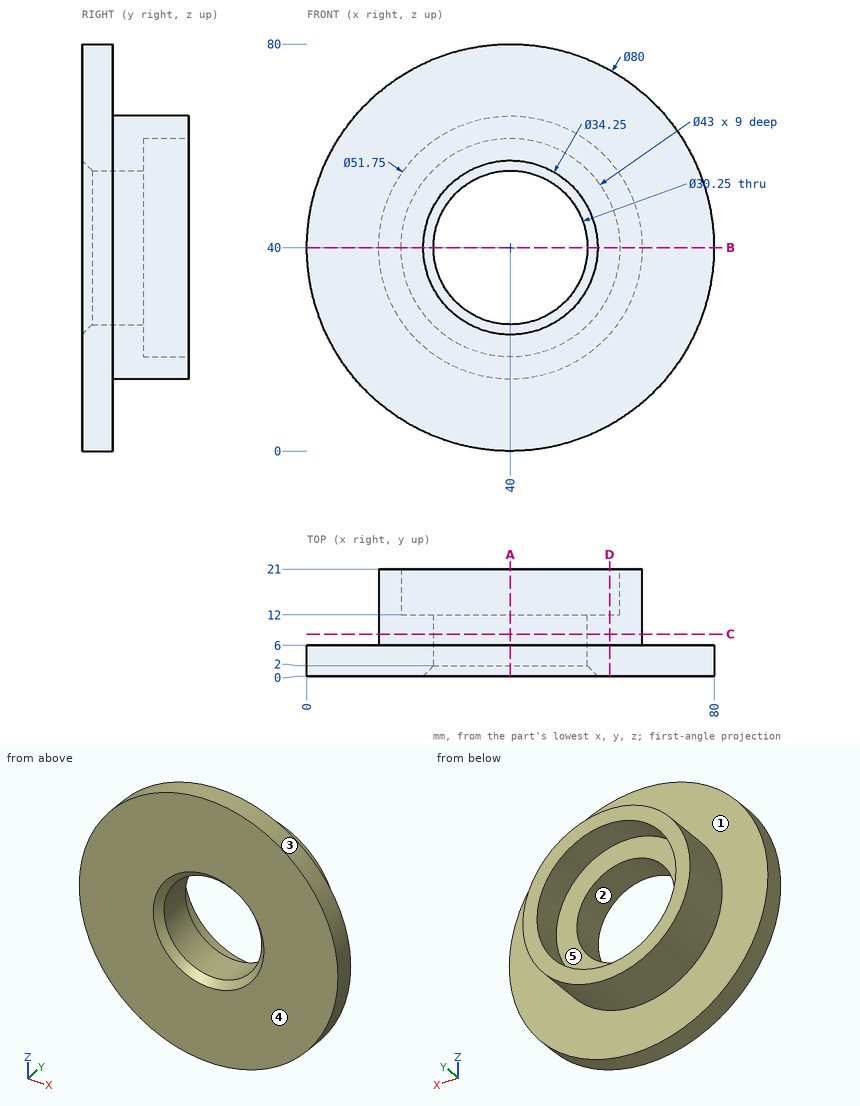
Print and shaded views of the part. All mm, measured from the part's lowest x, y and z. A direction names the side the tool comes from. Round coordinates to 2 decimals unless told otherwise and drop trailing zeros. Order: outer loops, then holes, each group sorted by start corner. A loop starts at its lowest first (then second) coordinate and runs counter-clockwise, first axis right, second up. Notation, with made-up numbers: (-27.75, 13.5) - (20.25, 13.5) arc R19 cw to (20.25, 48.5) - close; hole circle Ø4 at (19.25, 9). An arc over 180 degrees is marked (long way). Use a Markdown table: item, result.
1) Flat gauge pins, fed straight in: pin 1 Ø3 at (x, y) = (39.5, 13.5) entering from +Z (3 decimals); pin 2 Ø1.5 at (x, y) = (22.5, 2.5) entering from -Z; pin 3 Ø2 at (x, y) = (50, 6) entering from -Z. Where does each tip first touch, or does it go through?
Recorded:
| item | result |
|---|---|
| pin 1 | stops at z = 65.875 |
| pin 2 | stops at z = 3.68 |
| pin 3 | stops at z = 1.03 |
2) Wall check: L1, parallel to Z at x = 40, y = 14.25 (3 decimals); L2, parallel to Z at x = 40, y = 5.5 (3 decimals); L3, parallel to X at y = 8.5, z = 49. Give the ranges that are in metal, low to high.
Recorded:
| item | result |
|---|---|
| L1 | z = 14.125 to 18.5, 61.5 to 65.875 |
| L2 | z = 0 to 24.875, 55.125 to 80 |
| L3 | x = 15.74 to 27.84, 52.16 to 64.26 |
3) Saw through at B-B on z = 40. Write the cut outline in (x, y) (3 decimals), and give its area (3 significant figures).
Recorded:
| item | result |
|---|---|
| outline | (0, 0) - (22.875, 0) - (24.875, 2) - (24.875, 12) - (18.5, 12) - (18.5, 21) - (14.125, 21) - (14.125, 6) - (0, 6) - close; (55.125, 2) - (57.125, 0) - (80, 0) - (80, 6) - (65.875, 6) - (65.875, 21) - (61.5, 21) - (61.5, 12) - (55.125, 12) - close |
| area | 502 mm² |
4) Pull direction Z, two halves, no side cores. Call the marked faces 1, 2 and 3: pulls with the +Z half, pulls with the -Z half, needs draft (parallel to the pull), parting line crosses it, or undercut.
Recorded:
| item | result |
|---|---|
| face 1 | needs draft |
| face 2 | undercut |
| face 3 | parting line crosses it |
5) Tool access for the marked faces 4 and 5: list every direction of +Z, -Z, +X, -X, +Y, -Y with a clear straight run to the whole face (end or side of a thin tool).
Recorded:
| item | result |
|---|---|
| face 4 | +Z, -Z, +X, -X, -Y |
| face 5 | +Y |
6) Saw through at C-C on y = 8.25. Write the cut outline in (x, z) (3 decimals).
Recorded:
| item | result |
|---|---|
| outline | circle Ø51.75 at (40, 40); hole circle Ø30.25 at (40, 40) |
7) Saw through at A-A on x = 40. Write the cut outline in (y, z) (3 decimals).
Recorded:
| item | result |
|---|---|
| outline | (0, 0) - (6, 0) - (6, 14.125) - (21, 14.125) - (21, 18.5) - (12, 18.5) - (12, 24.875) - (2, 24.875) - (0, 22.875) - close; (0, 57.125) - (2, 55.125) - (12, 55.125) - (12, 61.5) - (21, 61.5) - (21, 65.875) - (6, 65.875) - (6, 80) - (0, 80) - close |
8) Saw through at D-D on x = 59.5. Write the cut outline in (y, z).
Recorded:
| item | result |
|---|---|
| outline | (0, 5.08) - (6, 5.08) - (6, 22.99) - (21, 22.99) - (21, 30.94) - (12, 30.94) - (12, 49.06) - (21, 49.06) - (21, 57.01) - (6, 57.01) - (6, 74.92) - (0, 74.92) - close |
